Build history of the part. All positions in model axes, mm. Round coordinates to 2 decimals unless told otherwise and drop trailing zeros. Loops run counter-clockwise (first coordinate to the right, second up) from the corner with the lowest first, then second, coordinate; pieces in that order, holes last. Notation, with made-up numbers: M 61.25,32 L 77.25,32 A20 cw 77.25,39 Z; hole C 65,64 d9. An arc over 180 degrees is marked long. One line per item, written item: value.
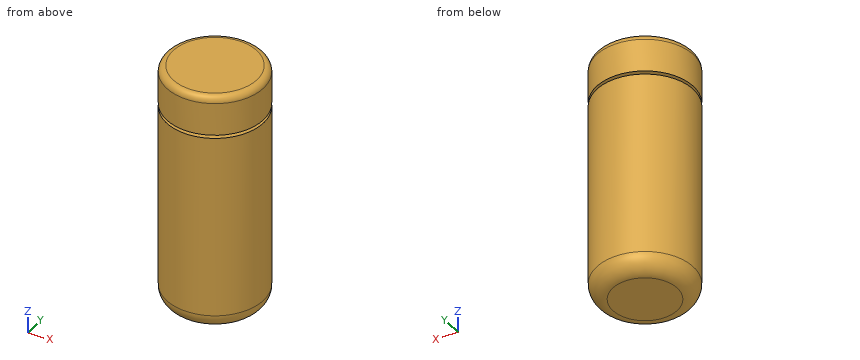
```python
from build123d import *

# Parameters (mm, degrees)
F0_R     = 15
F1_DEPTH = 75
F2_R     = 5
F3_R     = 2
F4_W     = 6.931401
F4_H     = 1


with BuildPart() as f1:
    # F0 (on Top) → F1 (new body)
    with BuildSketch(Plane.XY):
        Circle(F0_R)
    extrude(amount=F1_DEPTH)

    # F2
    f2_edges = [f1.edges().sort_by_distance(p)[0] for p in [
        (-15, 0, 0),
    ]]
    fillet(f2_edges, radius=F2_R)

    # F3
    f3_edges = [f1.edges().sort_by_distance(p)[0] for p in [
        (-15, 0, 75),
    ]]
    fillet(f3_edges, radius=F3_R)

    # F4 (on Right) → F5 (revolve, cut)
    with BuildSketch(Plane.YZ):
        with Locations((15.878135, 62.361921)):
            Rectangle(F4_W, F4_H)
    revolve(axis=Axis((0, 0, 55.164355), (0, 0, 1)), mode=Mode.SUBTRACT)


solid = f1.part
```
Item 1: Wall check: line 1 along Y through (x, z) = (-0.5, 57); line 2 along Z through (x, y) = (-7, 10.5); line 3 along X through (y, z) = (-2.75, 48). Give the ranges that are in metal, low to high.
Check values:
line 1: y = -14.99 to 14.99
line 2: z = 0.74 to 61.86, 62.86 to 75
line 3: x = -14.75 to 14.75
Item 2: Drop flat-ended pins along their axis: P1, Ø8, axis at x = -8, z = 29, coming from the +Y side; P2, Ø3, axis at x = 3.5, z = 58, coming from the +Y side; P3, Ø10, axis at x = 6.5, z = 67.5, coming from the -Y side. Give the stop position or say it passes through.
Check values:
P1: stops at y = 14.46
P2: stops at y = 14.87
P3: stops at y = -14.92
Item 3: Slice it at A-A, the plane z = 33.5. Give the cut face in (x, y).
Check values:
outline: C 0,0 d30
